from build123d import *

# Parameters (mm, degrees)
BOSS_EXTRUDE1_DEPTH     = 5
SKETCH2_R               = 2
CUT_EXTRUDE1_DEPTH      = 5
SKETCH4_R               = 3
CUT_EXTRUDE2_DEPTH      = 1.5
SKETCH25_R              = 2
CUT_EXTRUDE3_DEPTH      = 2
SKETCH19_R              = 2
CUT_EXTRUDE4_DEPTH      = 3
SKETCH26_W              = 14.53085056
SKETCH26_H              = 1
CUT_EXTRUDE5_DEPTH      = 2
CUT_EXTRUDE5_DEPTH_BACK = 2


with BuildPart() as part:
    # Sketch1 → Boss-Extrude1 (new body)
    with BuildSketch(Plane(origin=(0, 0, 0), x_dir=(1, 0, 0), z_dir=(0, 1, 0))):
        Polygon((9.270509831, -12.759762125), (15, -4.873795443), (15, 4.873795443), (9.270509831, 12.759762125), (0, 15.771933364), (-9.270509831, 12.759762125), (-15, 4.873795443), (-15, -4.873795443), (-9.270509831, -12.759762125), (0, -15.771933364), align=None)
    extrude(amount=BOSS_EXTRUDE1_DEPTH)

    # Sketch2 → Cut-Extrude1 (cut)
    with BuildSketch(Plane(origin=(0, 5, 0), x_dir=(1, 0, 0), z_dir=(0, 1, 0))):
        Circle(SKETCH2_R)
    extrude(amount=-CUT_EXTRUDE1_DEPTH, mode=Mode.SUBTRACT)

    # Sketch4 → Cut-Extrude2 (cut)
    with BuildSketch(Plane.XZ):
        Circle(SKETCH4_R)
    extrude(amount=-CUT_EXTRUDE2_DEPTH, mode=Mode.SUBTRACT)

    # Sketch25 → Cut-Extrude3 (cut)
    with BuildSketch(Plane(origin=(0, 5, 0), x_dir=(1, 0, 0), z_dir=(0, 1, 0))):
        with Locations((8.090169944, 5.877852523)):
            Circle(SKETCH25_R)
    extrude(amount=-CUT_EXTRUDE3_DEPTH, mode=Mode.SUBTRACT)

    # Sketch19 → Cut-Extrude4 (cut)
    with BuildSketch(Plane.XZ):
        with Locations((12.360679775, 0)):
            Circle(SKETCH19_R)
        with Locations((3.819660113, -11.755705046)):
            Circle(SKETCH19_R)
    extrude(amount=-CUT_EXTRUDE4_DEPTH, mode=Mode.SUBTRACT)

    # Sketch26 → Cut-Extrude5 (cut, two sides)
    with BuildSketch(Plane(origin=(8.090169944, 0, -5.877852523), x_dir=(-0.587785252, 0, -0.809016994), z_dir=(-0.809016994, 0, 0.587785252))) as cut_extrude5_sk:
        with Locations((0, -3)):
            Rectangle(SKETCH26_W, SKETCH26_H)
    extrude(amount=CUT_EXTRUDE5_DEPTH, mode=Mode.SUBTRACT)
    extrude(cut_extrude5_sk.sketch, amount=-CUT_EXTRUDE5_DEPTH_BACK, mode=Mode.SUBTRACT)


solid = part.part
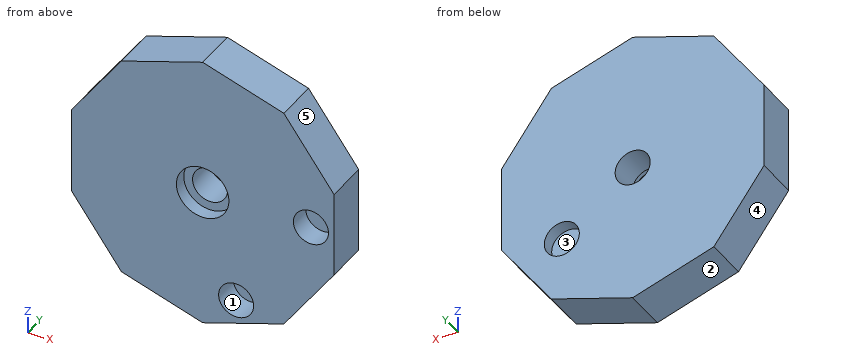
Read the model definition and answer for the solid it produces. Units are mm, in the model's axes. Face numbers are marked on the shaded views. A direction names the side the tool comes from. Coordinates: 2 decimals unless noted, no trailing zeros. Write each loop counter-clockwise with the first axis right and the second up, starting at its lowest first coordinate (ties: lowest second). Pieces come first, ordered by that corner, then holes. Notation, with made-up numbers: M 24,47 L 63,47 A24 cw 63,74 Z; hole C 48,53.5 d7. An arc over 180 degrees is marked long. Use a Markdown table: item, result.
Q1. Which of the six approach directions +Z, -Z, +X, -X, +Y, -Y give full straight-line access (tool end or side, diameter ignored) to the marked faces 1 and 2?
Answer block:
| item | result |
|---|---|
| face 1 | -Y |
| face 2 | -Z, -X, +Y, -Y |
Q2. Straight lines are drawn through the part: L1, parallel to X at y = 3.2, z = 0; L2, parallel to Y at x = 6, z = -9.5; L3, parallel to Z at x = 2.5, y = 1.05. For each, find the intervals that lie inside material, in ascending order. Write a range as [from, to].
Answer block:
| item | result |
|---|---|
| L1 | x = [-15, -2], [2, 9.89], [12.36, 15] |
| L2 | y = [0, 2.5], [3.5, 5] |
| L3 | z = [-14.96, -13.26], [-10.25, -1.66], [1.66, 14.96] |
Q3. Determine the mould class of the marked faces 3, 4 and 5 for opening direction X: released by +X, released by -X, zero draft, split by the parting line, or undercut.
Answer block:
| item | result |
|---|---|
| face 3 | undercut |
| face 4 | released by -X |
| face 5 | released by +X |
Q4. The part is cut by section B-B, the plane y = 4.1. Write down the section's boundary in (x, z), then the cut area to 3 significant figures.
Answer block:
| item | result |
|---|---|
| outline | M -15,-4.87 L -9.27,-12.76 L 0,-15.77 L 9.27,-12.76 L 15,-4.87 L 15,4.87 L 9.27,12.76 L 0,15.77 L -9.27,12.76 L -15,4.87 Z; hole C 0,0 d4; hole C 8.09,-5.88 d4 |
| area | 706 mm2 |
Q5. The part is cut by section A-A, the plane x = 0.5. Write down the section's boundary in (y, z), then the cut area to 3 significant figures.
Answer block:
| item | result |
|---|---|
| outline | M 0,-15.61 L 5,-15.61 L 5,-1.94 L 1.5,-1.94 L 1.5,-2.96 L 0,-2.96 Z; M 0,2.96 L 1.5,2.96 L 1.5,1.94 L 5,1.94 L 5,15.61 L 0,15.61 Z |
| area | 134 mm2 |
Q6. The part is cut by section D-D, the plane y = 0.9. Write down the section's boundary in (x, z), then the cut area to 3 significant figures.
Answer block:
| item | result |
|---|---|
| outline | M -15,-4.87 L -9.27,-12.76 L 0,-15.77 L 9.27,-12.76 L 15,-4.87 L 15,4.87 L 9.27,12.76 L 0,15.77 L -9.27,12.76 L -15,4.87 Z; hole C 0,0 d6; hole C 3.82,-11.76 d4; hole C 12.36,0 d4 |
| area | 678 mm2 |
Q7. The part is cut by section C-C, the plane z = 0. Write down the section's boundary in (x, y).
Answer block:
| item | result |
|---|---|
| outline | M -15,0 L -3,0 L -3,1.5 L -2,1.5 L -2,5 L -15,5 Z; M 2,1.5 L 3,1.5 L 3,0 L 10.36,0 L 10.36,2.5 L 9.89,2.5 L 9.89,3.5 L 12.36,3.5 L 12.36,3 L 14.36,3 L 14.36,0 L 15,0 L 15,5 L 2,5 Z |
Q8. Each of these flat-tipped pins is pushed along its axis until it touches: pin 1 Ø2.5 at (x, z) = (8.09, -5.88) entering from +Y; pin 2 Ø1.5 at (y, z) = (2.5, -7.5) entering from +X. Where does it stop, or does it pass through?
Answer block:
| item | result |
|---|---|
| pin 1 | stops at y = 2.5 |
| pin 2 | stops at x = 13.64 |
